Part print with two shaded views. Sizes in mm from the minimum x, y, z corner. A direction names the side the tool comes from. Round coordinates to 2 decimals unless told otherwise and drop trailing zeros. Order: outer loops, then holes, each group sorted by start corner. A loop starts at its lowest first (then second) coordinate and runs counter-clockwise, first axis right, second up. Notation, with made-up numbers: (72, 38) -> (91, 38) arc R14 cw to (91, 51) -> close; hole circle Ø4 at (17.5, 12). An arc over 180 degrees is marked (long way). Answer as a JSON object with one key per item and string values.
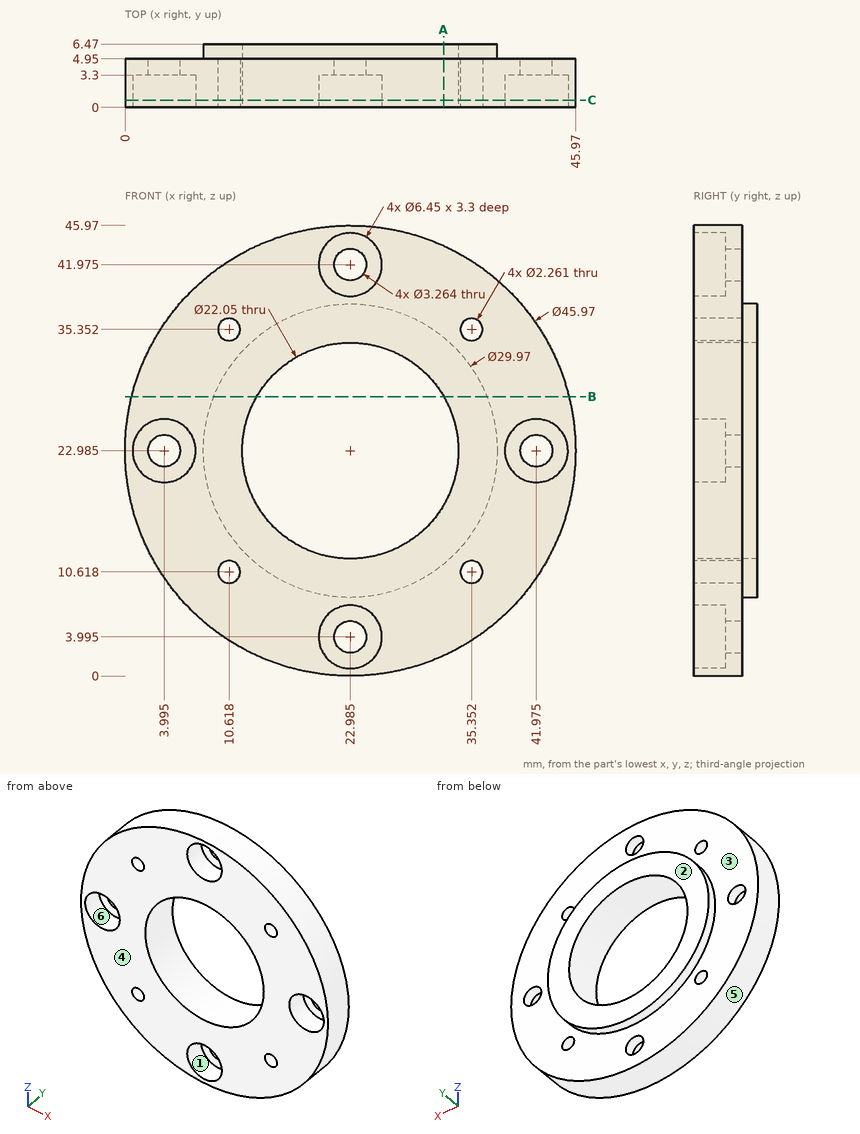
1) Flat gauge pins, fed straight in: pin 1 Ø4 at (x, z) = (22.985, 41.975) entering from -Y; pin 2 Ø8 at (x, z) = (26, 19.5) entering from +Y; pin 3 Ø1.5 at (x, y) = (28.5, 5) entering from -Z. Where does each tip first touch, or does it go through?
Checked values:
{"pin 1": "stops at y = 3.3", "pin 2": "passes through", "pin 3": "stops at z = 0.5"}
2) Probe L1, parallel to X at y = 5, z = 32 (1 decimal); L2, parallel to Z at x = 22.5, y = 1.25 (1 decimal); L3, parallel to X at y = 0.5, z = 5.5 (1 decimal). List the from-to ranges inside material, lowest first. Write a range as from..to.
Checked values:
{"L1": "x = 11..16.6, 29.3..35", "L2": "z = 0..0.8, 7.2..12, 34..38.8, 45.2..46", "L3": "x = 8.1..20.1, 25.8..37.9"}
3) Pull direction X, two halves, no side cores. Call the marked faces 4, 5 and 6: pulls with the +X half, pulls with the -X half, needs draft (parallel to the pull), parting line crosses it, or undercut.
Checked values:
{"face 4": "needs draft", "face 5": "parting line crosses it", "face 6": "undercut"}
4) Cut at A-A, the plane x = 32.5. Give the cut face in (y, z).
Checked values:
{"outline": "(0, 2.06) -> (4.95, 2.06) -> (4.95, 11.41) -> (6.47, 11.41) -> (6.47, 17.42) -> (0, 17.42) -> close; (0, 28.55) -> (6.47, 28.55) -> (6.47, 34.56) -> (4.95, 34.56) -> (4.95, 43.91) -> (0, 43.91) -> close"}
5) Cut at B-B, the plane z = 28.5. Give the cut face in (x, y), plus the area to 3 significant figures.
Checked values:
{"outline": "(0.67, 0) -> (13.44, 0) -> (13.44, 6.47) -> (9.05, 6.47) -> (9.05, 4.95) -> (0.67, 4.95) -> close; (32.53, 0) -> (45.3, 0) -> (45.3, 4.95) -> (36.92, 4.95) -> (36.92, 6.47) -> (32.53, 6.47) -> close", "area": "140 mm²"}
6) Which spindle directions (+Z, -Z, +X, -X, +Y, -Y) get a long thin tool onto all of the face, cutting with end or side? Do the marked faces 1, 2 and 3. Say none if no direction does.
Checked values:
{"face 1": "-Y", "face 2": "+Z, -Z, +X, -X, +Y", "face 3": "+Y"}
7) Cut at C-C, the plane y = 0.75. Count the separate pieces of the cut face and the enclosed holes in it, plus the area to 3 significant figures.
Checked values:
{"separate pieces": "1", "enclosed holes": "9", "area": "1,130 mm²"}
